Source: CAD feature listing. Evaluate the final solid. Frame: model axes, mm. Face numbers are marked on the shaded views. Give positions to 0.01 mm unless a question says otherwise; leave off trailing zeros. Loops run counter-clockwise (first coordinate to the right, second up) from the corner with the lowest first, then second, coordinate; pieces in that order, holes last. Notation, with made-up numbers: (54.5, -21) - (97.5, -21) arc R18 ccw to (97.5, -9) - close; hole circle Ø1 at (42, -12). An arc over 180 degrees is marked (long way). Write each question's results on one line, items separated by ' | '. Start each with the question number.
(1) Material intervals for line 1 along Z through (x, y) = (23.5, 4); line 2 along Z through (x, y) = (11.5, -2.25); line 3 along Y through (x, z) = (28, -23.5), sorted ascending. Write a range as [from, to].
(2) Pull-direction query (Z, two-part tool) for the marked faces 1, 2 and 3; classes: pulls with the +Z half, pulls with the -Z half, needs draft (parallel to the pull), parting line crosses it, or undercut.
(3) Cut plane C-C on x = 28. Return the cut outline in (y, z).
(4) Cut plane A-A on x = 12.5. Return the cut outline in (y, z), then the cut area to 3 significant figures.
(5) Cut plane B-B on z = 0. Return the cut outline in (x, y), then the cut area to 3 significant figures.
(6) Contact query for flat-ended pins moving along their axis: pin 1 (12 mm diameter, centred on x = 20.5, z = 28, fed in from +Y); pin 2 (1 mm diameter, centred on x = 17, y = 2.5, fed in from -Z); pin 3 (2 mm diameter, centred on x = 15.5, y = -4, fed in from -Z). Output: stop coordinate, or through.
(7) Cut plane D-D on y = -5.75. Return the cut outline in (x, z).
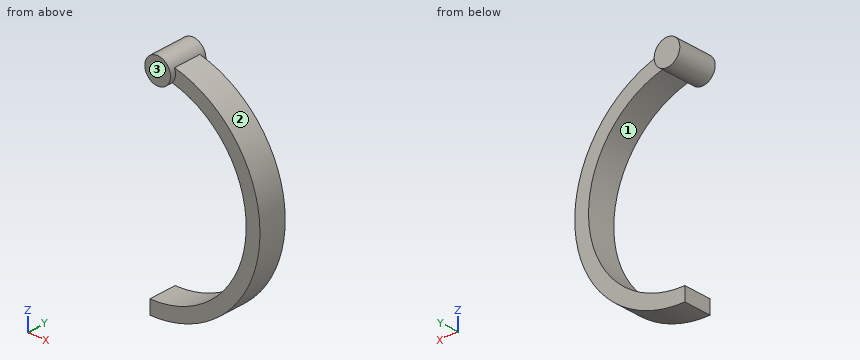
from build123d import *

# Parameters (mm, degrees)
EXTRUDE_2_DEPTH      = 7
EXTRUDE_2_DEPTH_BACK = 7
SKETCH_2_R           = 4.665046409
EXTRUDE_3_DEPTH      = 5
EXTRUDE_3_DEPTH_BACK = 5


with BuildPart() as part:
    # Sketch 2 → Extrude 2 (new, two sides: drawn at the far end of the back side and taken through both)
    with BuildSketch(Plane(origin=(0, 0, 0), x_dir=(1, 0, 0), z_dir=(0, 1, 0)).offset(-EXTRUDE_2_DEPTH_BACK)):
        with Locations(Location((4.665046409, -37.208699816, 0), (0, 0, 270))):
            Circle(SKETCH_2_R)
    extrude(amount=EXTRUDE_2_DEPTH + EXTRUDE_2_DEPTH_BACK)

    # Sketch 1 → Extrude 3 (add, two sides: drawn at the far end of the back side and taken through both)
    with BuildSketch(Plane(origin=(0, 0, 0), x_dir=(1, 0, 0), z_dir=(0, 1, 0)).offset(-EXTRUDE_3_DEPTH_BACK)):
        with BuildLine():
            Line((0, 35), (0, 40))
            ThreePointArc((0, 40), (39.743847013, 4.519582352), (8.981279477, -38.978668768))
            ThreePointArc((8.981279477, -38.978668768), (9.256967162, -36.385947248), (8.098232861, -34.050236776))
            ThreePointArc((8.098232861, -34.050236776), (34.761748281, 4.076868457), (0, 35))
        make_face()
    extrude(amount=EXTRUDE_3_DEPTH + EXTRUDE_3_DEPTH_BACK)


solid = part.part
Ans:
1) line 1: [-32.37, -25.94], [25.94, 32.37] | line 2: [-38.31, -33.06], [33.06, 38.31] | line 3: [-5, 5]
2) face 1: undercut | face 2: parting line crosses it | face 3: needs draft
3) outline: (-5, -28.57) - (5, -28.57) - (5, -21) - (-5, -21) - close; (-5, 21) - (5, 21) - (5, 28.57) - (-5, 28.57) - close
4) outline: (-5, -38) - (5, -38) - (5, -32.69) - (-5, -32.69) - close; (-5, 32.69) - (5, 32.69) - (5, 38) - (-5, 38) - close | area: 106 mm^2
5) outline: (35, -5) - (40, -5) - (40, 5) - (35, 5) - close | area: 50.0 mm^2
6) pin 1: y = 5 | pin 2: z = -36.44 | pin 3: z = -37.28
7) outline: circle Ø9.33 at (4.67, 37.21)
